For this review, use the dimensioned drawing (mm, ordinates from the lowest corner) and the shaded views. A direction names the side the tool comes from. Round coordinates to 2 decimals unless told otherwise and drop trailing zeros. Write each loop counter-clockwise with the first axis right and the second up, starting at its lowest first coordinate (ties: lowest second). Pieces come first, ordered by that corner, then holes. Notation, with made-up numbers: (29.5, -32.75) - (48.5, -32.75) arc R14 cw to (48.5, -20.75) - close; hole circle Ø3 at (28, 8). An arc over 180 degrees is marked (long way). Write each question's results on one line, items separated by ' | '.
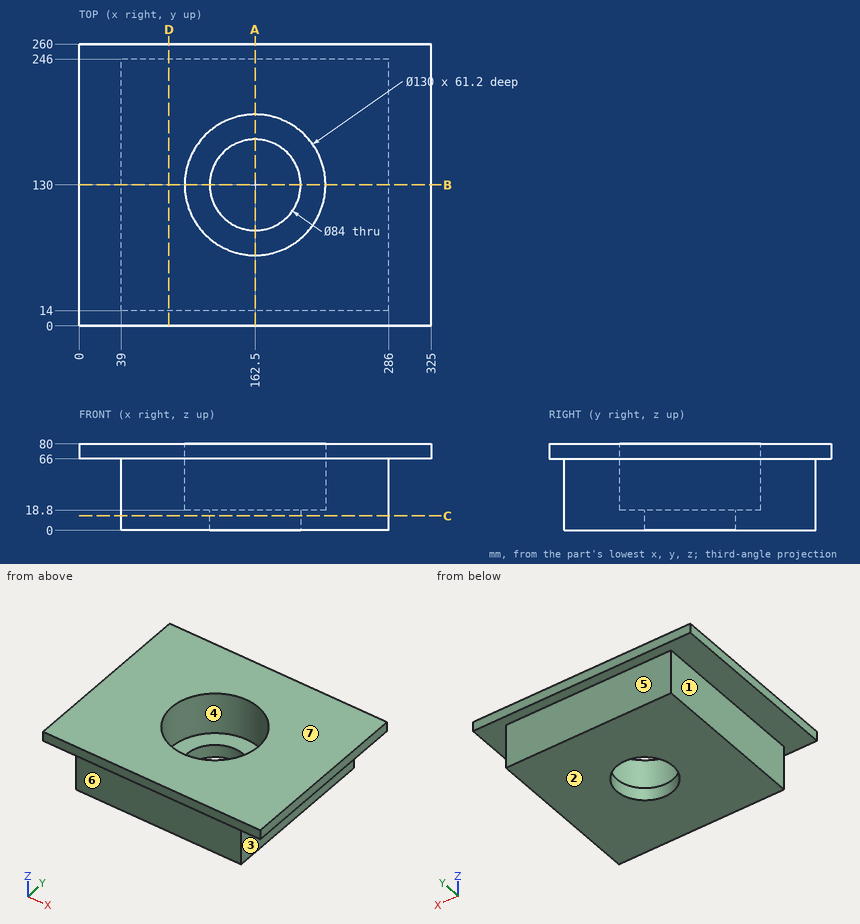
Q1. Insertion check: P1, Ø1, axis at x = 259, z = 16.5, coming from the -Y side; P2, Ø20, axis at x = 218, z = 24, coming from the +Y side; P3, Ø20, axis at y = 109, z = 37.5, coming from the -X side. Each pin has a flat end and moves straight along its axis. Give the tip position at first contact, or say it passes through.
Evaluation:
P1: stops at y = 14 | P2: stops at y = 246 | P3: stops at x = 39
Q2. We need section A-A (x = 162.5). State the section outline as (y, z) points.
Evaluation:
outline: (0, 66) - (14, 66) - (14, 0) - (88, 0) - (88, 18.8) - (65, 18.8) - (65, 80) - (0, 80) - close; (172, 0) - (246, 0) - (246, 66) - (260, 66) - (260, 80) - (195, 80) - (195, 18.8) - (172, 18.8) - close
Q3. Tool access review of the marked faces 1, 2 and 3: name each direction out of +Z, -Z, +X, -X, +Y, -Y from which nothing blocks a thin tool from reaching the whole face with its end or side.
Evaluation:
face 1: -Z, -X, +Y, -Y | face 2: -Z, +X, -X, +Y, -Y | face 3: -Z, +X, +Y, -Y
Q4. We need section C-C (z = 13.5). State the section outline as (x, y) points.
Evaluation:
outline: (39, 14) - (286, 14) - (286, 246) - (39, 246) - close; hole circle Ø84 at (162.5, 130)
Q5. We need section D-D (x = 83). State the section outline as (y, z) points, plus the area to 3 significant figures.
Evaluation:
outline: (0, 66) - (14, 66) - (14, 0) - (246, 0) - (246, 66) - (260, 66) - (260, 80) - (0, 80) - close | area: 19,000 mm^2
Q6. The part is to be moulded in two halves that separate along Y. For the marked faces 4, 5, 6 and 7, say which applies: released by +Y, released by -Y, zero draft, split by the parting line, or undercut.
Evaluation:
face 4: undercut | face 5: released by +Y | face 6: released by -Y | face 7: zero draft
Q7. For probe 1 along Y at (x, z) = (162.5, 61.5); probe 2 along Y at (x, z) = (159.5, 74.5); probe 3 along X at (y, z) = (20, 48.5), list the stretches that pass through material, from the lowest coordinate up.
Evaluation:
probe 1: y = 14 to 65, 195 to 246 | probe 2: y = 0 to 65.07, 194.93 to 260 | probe 3: x = 39 to 286
Q8. We need section B-B (y = 130). State the section outline as (x, z) points.
Evaluation:
outline: (0, 66) - (39, 66) - (39, 0) - (120.5, 0) - (120.5, 18.8) - (97.5, 18.8) - (97.5, 80) - (0, 80) - close; (204.5, 0) - (286, 0) - (286, 66) - (325, 66) - (325, 80) - (227.5, 80) - (227.5, 18.8) - (204.5, 18.8) - close
